Design review of the part built by this model. Coordinates are the model's own, in mm. A direction names the side the tool comes from. Coordinates: 2 decimals unless noted, no trailing zeros. Write each loop counter-clockwise with the first axis right and the second up, starting at its lowest first coordinate (ties: lowest second). Pieces come first, ordered by that corner, then holes. Notation, with made-up numbers: (68, 45.25) -> (123, 45.25) arc R19 cw to (123, 65.25) -> close; hole circle Ø5 at (13.25, -10). An arc over 180 degrees is marked (long way). Answer in a Markdown table with one row per item. Add a question column.
Item 1: Clearance check with flat-ended pins moving along their axes: P1, Ø16.5, axis at x = -1, y = 17, coming from the +Z side; P2, Ø6.5, axis at x = -5, z = 11.5, coming from the -Y side; P3, Ø8, axis at y = 18.5, z = 8, coming from the -X side. State where each tip first meets the part, or that it passes through.
Item 2: Take a section at C-C, the plane y = 33.5. Write out the cut boundary in (x, z), and give its area (3 significant figures).
Item 3: Draft analysis for pull direction Y (two halves, no side actions). For faces 6 (the face through (16.35, 20.37, 3.55)), 7 (the face through (16.5, 14, 3)), 8 (the face through (16.199, 35.285, 11.056)), state which applies: released by +Y, released by -Y, zero draft, split by the parting line, or undercut.
Item 4: Take a section at D-D, the plane z = 2.25. Give the number of separate pieces and of enclosed holes in the cut face, and give its area (3 significant figures).
Item 5: Take a section at B-B, the plane x = -5. Write out the cut boundary in (y, z), and give its area (3 significant figures).
Item 6: For faces 1 (the face through (0.1, 29.5, 7.5)), 2 (the face through (16.357, 26.093, 3.549)), 3 (the face through (3, 31, 0)), 4 (the face through (0, 45, 15)), 5 (the face through (14.785, 35.301, 11.056)), list the 3-axis set-ups (+Z, -Z, +X, -X, +Y, -Y) from which the entire face can be reached by the end or side of a thin tool; tool diameter is ignored.
Item 7: To check wall thickness, follow line 1 (Y direction, x = 12.5, z = 2.25); line 2 (Z direction, x = 11.5, y = 10.5); line 3 (X direction, y = 39, z = 1). State the ranges of each line that lie inside material, in increasing order.
from build123d import *

# Parameters (mm, degrees)
BOSS_EXTRUDE1_DEPTH = 7
BOSS_EXTRUDE2_DEPTH = 8
FILLET1_R           = 3.5
BOSS_EXTRUDE3_DEPTH = 1
FILLET5_R           = 0.5
SKETCH3_R           = 3.6
SKETCH3_R_2         = 3.55
CUT_EXTRUDE2_DEPTH  = 12
FILLET7_R           = 4
FILLET8_R           = 1
SKETCH5_R           = 1.65
SKETCH5_R_2         = 1.6
CUT_EXTRUDE3_DEPTH  = 51.450470761
FILLET12_R          = 4


# Some blends are built 0.0001 mm under size
with BuildPart() as part:
    # Sketch1 → Boss-Extrude1 (new body)
    with BuildSketch(Plane.XY):
        with BuildLine():
            Line((16.5, 47), (-16.5, 47))
            Line((-16.5, 47), (-16.5, 28))
            Line((-16.5, 28), (3.206829084, 10.522178825))
            ThreePointArc((3.206829084, 10.522178825), (7.298815617, 8.229659203), (10.063744764, 4.440837907))
            Line((10.063744764, 4.440837907), (16.5, -1.267422796))
            Line((16.5, -1.267422796), (16.5, 47))
        make_face()
    extrude(amount=BOSS_EXTRUDE1_DEPTH)

    # Sketch2 → Boss-Extrude2 (add)
    with BuildSketch(Plane.XY.offset(7)):
        Polygon((-16.5, 35), (-16.5, 47), (16.5, 47), (16.5, 35), (14.5, 35), (14.5, 44), (-14.5, 44), (-14.5, 35), align=None)
    extrude(amount=BOSS_EXTRUDE2_DEPTH)

    # Fillet1
    fillet1_edges = [part.edges().sort_by_distance(p)[0] for p in [
        (-14.5, 44, 11),
        (14.5, 44, 11),
    ]]
    fillet(fillet1_edges, radius=FILLET1_R)

    # Sketch4 → Boss-Extrude3 (add)
    with BuildSketch(Plane.XY.offset(7)):
        with BuildLine():
            ThreePointArc((7.763157895, 28.460206948), (0, 29.5), (-7.763157895, 28.460206948))
            Line((-7.763157895, 28.460206948), (-7.5, 27.49545417))
            ThreePointArc((-7.5, 27.49545417), (0, 28.5), (7.5, 27.49545417))
            Line((7.5, 27.49545417), (7.763157895, 28.460206948))
        make_face()
    extrude(amount=BOSS_EXTRUDE3_DEPTH)

    # Fillet5
    fillet5_edges = [part.edges().sort_by_distance(p)[0] for p in [
        (7.763157895, 28.460206948, 7.5),
        (7.5, 27.49545417, 7.5),
        (-7.763157895, 28.460206948, 7.5),
        (-7.5, 27.49545417, 7.5),
    ]]
    fillet(fillet5_edges, radius=FILLET5_R - 0.0001)  # a hair under: the kernel refuses the full size

    # Sketch3 → Cut-Extrude2 (cut)
    with BuildSketch(Plane(origin=(0, 0, 0), x_dir=(-1, 0, 0), z_dir=(0, 0, -1))):
        with Locations((-19, 23.216373532)):
            Circle(SKETCH3_R)
        with Locations((19, 23.216373532)):
            Circle(SKETCH3_R_2)
    extrude(amount=-CUT_EXTRUDE2_DEPTH, mode=Mode.SUBTRACT)

    # Fillet7
    # the kernel refuses this fillet: 4 mm, written as the material it takes off along each edge
    with BuildSketch(Plane(origin=(3.206829084, 10.522178825, -2.00647278), x_dir=(0.9469871930704206, -0.3212713123834835, 0), z_dir=(0, 0, 1))) as fillet7_piece_1:
        with BuildLine():
            CenterArc((0.812259209, 3.998047556), FILLET7_R, 247.170276445, 21.039469781)
            Line((-0.739715882, 0.311399578), (0, 0))
            ThreePointArc((0, 0), (0.343648127, 0.005369221), (0.687296254, 0))
        make_face()
    extrude(amount=11.012945561, mode=Mode.SUBTRACT)
    with BuildSketch(Plane(origin=(-16.5, 28, -4.497372603), x_dir=(0.7481508366108257, -0.6635286924304943, 0), z_dir=(0, 0, 1))) as fillet7_piece_2:
        with BuildLine():
            CenterArc((FILLET7_R * 0.449737260328, FILLET7_R), FILLET7_R, 221.569549454, 48.430450546)
            Line((-FILLET7_R * 0.298413576283, FILLET7_R * 0.33647130757), (0, 0))
            Line((0, 0), (FILLET7_R * 0.449737260328, 0))
        make_face()
    extrude(amount=15.994745207, mode=Mode.SUBTRACT)
    with BuildSketch(Plane(origin=(16.5, -1.267422796, -22.201864002), x_dir=(0, 1, 0), z_dir=(0, 0, 1))) as fillet7_piece_3:
        with BuildLine():
            CenterArc((8.880745601, 4), FILLET7_R, 142.478159004, 127.521840996)
            Line((5.708260703, 6.436255236), (0, 0))
            Line((0, 0), (8.880745601, 0))
        make_face()
    extrude(amount=51.403728005, mode=Mode.SUBTRACT)
    with BuildSketch(Plane(origin=(16.5, 25.806740302, 10.36976741), x_dir=(0, 1, 0), z_dir=(0, 0, -1))) as fillet7_piece_4:
        with BuildLine():
            CenterArc((1.347906964, -4), FILLET7_R, 90, 31.211180498)
            ThreePointArc((-0.724868685, -0.578947368), (-0.343707491, -0.312920562), (0, 0))
            Line((0, 0), (1.347906964, 0))
        make_face()
    extrude(amount=13.739534821, mode=Mode.SUBTRACT)
    with BuildSketch(Plane(origin=(16.5, 20.626006763, 10.36976741), x_dir=(-0.6240720217299989, 0.7813668227496173, 0), z_dir=(0, 0, -1))) as fillet7_piece_5:
        with BuildLine():
            CenterArc((1.443078305, -3.966658315), FILLET7_R, 97.402928186, 31.211180498)
            Line((-1.053209782, -0.841191024), (0, 0))
            ThreePointArc((0, 0), (0.463846598, -0.030007516), (0.927693196, 0))
        make_face()
    extrude(amount=13.739534821, mode=Mode.SUBTRACT)

    # Fillet8
    fillet8_edges = [part.edges().sort_by_distance(p)[0] for p in [
        (-16.5, 47, 7.5),
        (16.5, 47, 7.5),
        (-16.5, 35, 11),
        (-14.5, 35, 11),
        (14.5, 35, 11),
        (16.5, 35, 11),
    ]]
    fillet(fillet8_edges, radius=FILLET8_R - 0.0001)  # a hair under: the kernel refuses the full size

    # Sketch5 → Cut-Extrude3 (cut, through all)
    with BuildSketch(Plane.XY.offset(7)):
        with Locations((-11, 40.5)):
            Circle(SKETCH5_R)
        with Locations((11, 40.5)):
            Circle(SKETCH5_R)
        with Locations((12.5, 8.291561976)):
            Circle(SKETCH5_R_2)
        with Locations((12.5, 20.487801249)):
            Circle(SKETCH5_R_2)
        with Locations((-5.294742993, 23.408667127)):
            Circle(SKETCH5_R_2)
    extrude(amount=-CUT_EXTRUDE3_DEPTH, mode=Mode.SUBTRACT)

    # Fillet12
    fillet12_edges = [part.edges().sort_by_distance(p)[0] for p in [
        (10.063744764, 4.440837907, 3.5),
    ]]
    fillet(fillet12_edges, radius=FILLET12_R - 0.0001)  # a hair under: the kernel refuses the full size


solid = part.part
Answers:
| question | item | result |
|---|---|---|
| 1 | P1 | stops at z = 7 |
| 1 | P2 | stops at y = 44 |
| 1 | P3 | stops at x = -10.16 |
| 2 | outline | (-16.5, 0) -> (16.5, 0) -> (16.5, 7) -> (-16.5, 7) -> close |
| 2 | area | 231 mm^2 |
| 3 | face 6 | undercut |
| 3 | face 7 | zero draft |
| 3 | face 8 | released by -Y |
| 4 | separate pieces | 1 |
| 4 | enclosed holes | 5 |
| 4 | area | 1,040 mm^2 |
| 5 | outline | (17.8, 0) -> (21.84, 0) -> (21.84, 7) -> (17.8, 7) -> close; (24.98, 0) -> (47, 0) -> (47, 15) -> (44, 15) -> (44, 7) -> (29.07, 7) -> (29.07, 8) -> (28.06, 8) -> (28.06, 7) -> (24.98, 7) -> close |
| 5 | area | 207 mm^2 |
| 6 | face 1 | +Z |
| 6 | face 2 | +Z, -Z, +X |
| 6 | face 3 | -Z, +X, -X, +Y, -Y |
| 6 | face 4 | +Z, +X, -X, +Y, -Y |
| 6 | face 5 | +Z, -Y |
| 7 | line 1 | y = 4.29 to 6.69, 9.89 to 18.89, 22.09 to 39.81, 41.19 to 47 |
| 7 | line 2 | z = 0 to 7 |
| 7 | line 3 | x = -16.5 to -11.69, -10.31 to 10.31, 11.69 to 16.5 |
